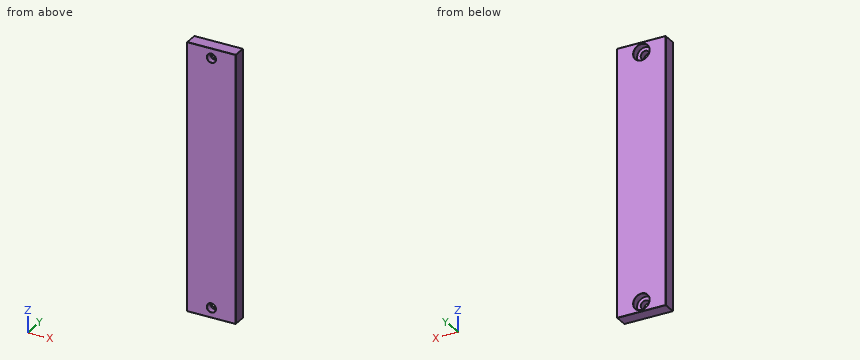
from build123d import *

# Parameters (mm, degrees)
SKETCH1_W           = 30
SKETCH1_H           = 165
SKETCH1_R           = 2.75
BOSS_EXTRUDE2_DEPTH = 8
SKETCH3_R           = 5
CUT_EXTRUDE1_DEPTH  = 4.2
CHAMFER1_SIZE       = 0.1


with BuildPart() as part:
    # Sketch1 → Boss-Extrude2 (new body)
    with BuildSketch(Plane(origin=(0, 0, 0), x_dir=(1, 0, 0), z_dir=(0, 1, 0))):
        Rectangle(SKETCH1_W, SKETCH1_H)
        with Locations((0, 76.5)):
            Circle(SKETCH1_R, mode=Mode.SUBTRACT)
        with Locations((0, -76.5)):
            Circle(SKETCH1_R, mode=Mode.SUBTRACT)
    extrude(amount=BOSS_EXTRUDE2_DEPTH)

    # Sketch3 → Cut-Extrude1 (cut)
    with BuildSketch(Plane(origin=(0, 8, 0), x_dir=(1, 0, 0), z_dir=(0, 1, 0))):
        with Locations((0, 76.5)):
            Circle(SKETCH3_R)
        with Locations((0, -76.5)):
            Circle(SKETCH3_R)
    extrude(amount=-CUT_EXTRUDE1_DEPTH, mode=Mode.SUBTRACT)

    # Chamfer1
    chamfer1_edges = [part.edges().sort_by_distance(p)[0] for p in [
        (-2.75, 0, -76.5),
        (-15, 8, 0),
        (-2.75, 0, 76.5),
        (0, 8, 82.5),
        (-5, 8, -76.5),
        (-5, 8, 76.5),
        (15, 8, 0),
        (0, 0, 82.5),
        (-15, 0, 0),
        (0, 0, -82.5),
        (15, 0, 0),
        (15, 4, 82.5),
        (-15, 4, 82.5),
        (-15, 4, -82.5),
        (15, 4, -82.5),
        (0, 8, -82.5),
    ]]
    chamfer(chamfer1_edges, length=CHAMFER1_SIZE)


solid = part.part
Source: CAD feature listing. Evaluate the final solid. Frame: model axes, mm. Coordinates: 2 decimals unless noted, no trailing zeros. Order: outer loops, then holes, each group sorted by start corner. A loop starts at its lowest first (then second) coordinate and runs counter-clockwise, first axis right, second up. Notation, with made-up numbers: M 21.25,64 L 55.25,64 A9 ccw 55.25,76 Z; hole C -39.5,-25.75 d1. An arc over 180 degrees is marked long. Write each question's results on one line, items separated by ' | '. Start each with the question number.
Item 1: Cut plane C-C (y = 5.25). Return loops of the section in (x, z), and give its area (3 significant figures).
Item 2: Line query: probe 1 along Z at (x, y) = (0, 6.9); probe 2 along Z at (x, y) = (0, 1); probe 3 along X at (y, z) = (5.4, 76.5). Output: solid intervals per line, ascending.
Item 3: Cut plane B-B (x = 0). Count the separate pieces of the cut face and the enclosed holes in it, and give its area (3 significant figures).
Item 4: Cut plane A-A (z = 76.5). Return loops of the section in (x, y), and give its area (3 significant figures).
Item 5: First-contact query: pin 1 Ø5 at (x, z) = (-0.5, -78) entering from +Y. Flat tip, straight axial feed; report the tip coordinate or a pass-through.
Checked values:
1) outline: M -15,-82.4 L -14.9,-82.5 L 14.9,-82.5 L 15,-82.4 L 15,82.4 L 14.9,82.5 L -14.9,82.5 L -15,82.4 Z; hole C 0,-76.5 d10; hole C 0,76.5 d10 | area: 4,790 mm2
2) probe 1: z = -82.5 to -81.5, -71.5 to 71.5, 81.5 to 82.5 | probe 2: z = -82.5 to -79.25, -73.75 to 73.75, 79.25 to 82.5 | probe 3: x = -15 to -5, 5 to 15
3) separate pieces: 3 | enclosed holes: 0 | area: 1,190 mm2
4) outline: M -15,0.1 L -14.9,0 L -2.85,0 L -2.75,0.1 L -2.75,3.8 L -5,3.8 L -5,7.9 L -5.1,8 L -14.9,8 L -15,7.9 Z; M 2.75,0.1 L 2.85,0 L 14.9,0 L 15,0.1 L 15,7.9 L 14.9,8 L 5.1,8 L 5,7.9 L 5,3.8 L 2.75,3.8 Z | area: 177 mm2
5) pin 1: stops at y = 3.8
